from build123d import *

# Parameters (mm, degrees)
F0_R     = 3.175
F0_R_2   = 12.7
F0_R_3   = 6.35
F1_DEPTH = 12.7


with BuildPart() as f1:
    # F0 (on Front) → F1 (new body)
    with BuildSketch(Plane.XZ):
        with BuildLine():
            ThreePointArc((-31.115, -6.985), (-26.175859, -4.939141), (-24.13, 0))
            ThreePointArc((-24.13, 0), (-26.175859, 4.939141), (-31.115, 6.985))
            ThreePointArc((-31.115, 6.985), (-38.1, 0), (-31.115, -6.985))
        make_face()
        with Locations((-31.115, 0)):
            Circle(F0_R, mode=Mode.SUBTRACT)
        with BuildLine():
            ThreePointArc((-31.115, 6.985), (-26.175859, 4.939141), (-24.13, 0))
            ThreePointArc((-24.13, 0), (-26.175859, -4.939141), (-31.115, -6.985))
            Line((-31.115, -6.985), (-6.985, -31.115))
            ThreePointArc((-6.985, -31.115), (0, -24.13), (6.985, -31.115))
            Line((6.985, -31.115), (31.115, -6.985))
            ThreePointArc((31.115, -6.985), (24.13, 0), (31.115, 6.985))
            Line((31.115, 6.985), (6.985, 31.115))
            ThreePointArc((6.985, 31.115), (0, 24.13), (-6.985, 31.115))
            Line((-6.985, 31.115), (-31.115, 6.985))
        make_face()
        Circle(F0_R_2, mode=Mode.SUBTRACT)
        with BuildLine():
            ThreePointArc((6.985, 31.115), (0, 38.1), (-6.985, 31.115))
            ThreePointArc((-6.985, 31.115), (0, 24.13), (6.985, 31.115))
        make_face()
        with Locations((0, 31.115)):
            Circle(F0_R, mode=Mode.SUBTRACT)
        with BuildLine():
            ThreePointArc((6.985, -31.115), (0, -24.13), (-6.985, -31.115))
            ThreePointArc((-6.985, -31.115), (0, -38.1), (6.985, -31.115))
        make_face()
        with Locations((0, -31.115)):
            Circle(F0_R, mode=Mode.SUBTRACT)
        with BuildLine():
            ThreePointArc((38.1, 0), (36.054141, 4.939141), (31.115, 6.985))
            ThreePointArc((31.115, 6.985), (24.13, 0), (31.115, -6.985))
            ThreePointArc((31.115, -6.985), (36.054141, -4.939141), (38.1, 0))
        make_face()
        with Locations((31.115, 0)):
            Circle(F0_R, mode=Mode.SUBTRACT)
        Circle(F0_R_2)
        Circle(F0_R_3, mode=Mode.SUBTRACT)
    extrude(amount=F1_DEPTH)


solid = f1.part
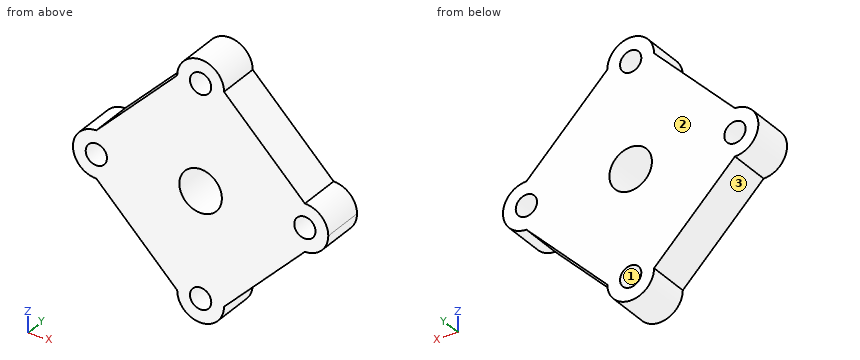
For this review, take the finished solid that the model builds, in its own axes (mm). Face numbers are marked on the shaded views. Give positions to 0.01 mm unless a question says otherwise; leave off trailing zeros. Loops run counter-clockwise (first coordinate to the right, second up) from the corner with the lowest first, then second, coordinate; pieces in that order, holes last.
Item 1: Take a section at A-A, the plane x = 0. State the section outline as (y, z) points, and give its area (3 significant figures).
Item 2: Take a section at B-B, the plane y = -2. State the section outline as (x, z) points (3 decimals), and give its area (3 significant figures).
Item 3: For line 1 along Z through (x, y) = (0, -7); line 2 along X through (y, z) = (-8.75, -33); line 3 along X through (y, z) = (-2.25, -32.5), list the stretches that pass through material, from the lowest coordinate up.
Item 4: Draft analysis for pull direction Z (two halves, no side actions). For the marked faces 1, 2 and 3, state which applies: +Z half, -Z half, draft (parallel to the pull), parting line (faces both ways), or undercut.
Item 5: Insertion check: pin 1 (4 mm diameter, centred on x = 10, y = -5.5, fed in from +Z); pin 2 (4 mm diameter, centred on y = -4.5, z = -18.5, fed in from -X); pin 3 (2 mm diameter, centred on y = -9.5, z = 10, fed in from -X). Each pin has a flat end and moves straight along its axis. Give the tip position at first contact, or say it passes through.
Item 6: Take a section at C-C, the plane z = -1.5. State the section outline as (x, y) points.
Item 7: Take a section at D-D, the plane x = -20.5. State the section outline as (y, z) points, and give its area (3 significant figures).
Calculated:
1. outline: (-12.7, -38.1) - (0, -38.1) - (0, -34.29) - (-12.7, -34.29) - close; (-12.7, -27.94) - (0, -27.94) - (0, -6.35) - (-12.7, -6.35) - close; (-12.7, 6.35) - (0, 6.35) - (0, 27.94) - (-12.7, 27.94) - close; (-12.7, 34.29) - (0, 34.29) - (0, 38.1) - (-12.7, 38.1) - close
1. area: 645 mm2
2. outline: (-31.115, -6.985) - (-6.985, -31.115) arc R6.985 ccw to (6.985, -31.115) - (31.115, -6.985) arc R6.985 ccw to (31.115, 6.985) - (6.985, 31.115) arc R6.985 ccw to (-6.985, 31.115) - (-31.115, 6.985) arc R6.985 ccw to start; hole circle Ø6.35 at (-31.115, 0); hole circle Ø12.7 at (0, 0); hole circle Ø6.35 at (0, -31.115); hole circle Ø6.35 at (0, 31.115); hole circle Ø6.35 at (31.115, 0)
2. area: 2,760 mm2
3. line 1: z = -38.1 to -34.29, -27.94 to -6.35, 6.35 to 27.94, 34.29 to 38.1
3. line 2: x = -6.73 to -2.55, 2.55 to 6.73
3. line 3: x = -6.85 to -2.86, 2.86 to 6.85
4. face 1: undercut
4. face 2: draft
4. face 3: -Z half
5. pin 1: stops at z = 30.1
5. pin 2: stops at x = -21.6
5. pin 3: stops at x = -29.1
6. outline: (-37.94, -12.7) - (-33.91, -12.7) - (-33.91, 0) - (-37.94, 0) - close; (-28.32, -12.7) - (-6.17, -12.7) - (-6.17, 0) - (-28.32, 0) - close; (6.17, -12.7) - (28.32, -12.7) - (28.32, 0) - (6.17, 0) - close; (33.91, -12.7) - (37.94, -12.7) - (37.94, 0) - (33.91, 0) - close
7. outline: (-12.7, -17.6) - (0, -17.6) - (0, 17.6) - (-12.7, 17.6) - close
7. area: 447 mm2
